Read the model definition and answer for the solid it produces. Units are mm, in the model's axes. A direction names the side the tool comes from. Coordinates: 2 decimals unless noted, no trailing zeros. Write each loop counter-clockwise with the first axis right and the second up, starting at its lowest first coordinate (ties: lowest second). Pieces come first, ordered by that corner, then holes. Notation, with made-up numbers: M 82.5,66.5 L 121.5,66.5 A18 ccw 121.5,78.5 Z; hole C 72.25,-20.5 d4. An arc over 180 degrees is marked long. Write item = value, one per line.
from build123d import *

# Parameters (mm, degrees)
BOSS_EXTRUDE1_DEPTH                           = 10
CBORE_FOR_M3_HEX_HEAD_MACHINE_SCREW3_AT_COUNT = 2
CBORE_FOR_M3_HEX_HEAD_MACHINE_SCREW3_AT_PITCH = 31.112698372
CBORE_FOR_M3_HEX_HEAD_MACHINE_SCREW3_2_COUNT  = 2
CBORE_FOR_M3_HEX_HEAD_MACHINE_SCREW3_2_PITCH  = 44


with BuildPart() as part:
    # Sketch1 → Boss-Extrude1 (new body)
    with BuildSketch(Plane.XY):
        with BuildLine():
            Line((-16.007810594, -4), (-21, -4))
            Line((-21, -4), (-21, 4))
            Line((-21, 4), (-16.007810594, 4))
            ThreePointArc((-16.007810594, 4), (0, 16.5), (16.007810594, 4))
            Line((16.007810594, 4), (24.677925359, 4))
            ThreePointArc((24.677925359, 4), (-25, 0), (24.677925359, -4))
            Line((24.677925359, -4), (16.007810594, -4))
            ThreePointArc((16.007810594, -4), (0, -16.5), (-16.007810594, -4))
        make_face()
    extrude(amount=BOSS_EXTRUDE1_DEPTH)

    # Sketch6 → CBORE for M3 Hex Head Machine Screw2 (revolve, cut)
    with BuildSketch(Plane(origin=(20.342867976, 24, 5), x_dir=(0, 0, 1), z_dir=(1, 0, 0))):
        Polygon((0, 0), (0, 49), (1.7, 49), (1.7, 17.3), (4.2, 17.3), (4.2, 0.025), (4.225, 0), align=None)
    revolve(axis=Axis((20.342867976, 30.35, 5), (0, -1, 0)), mode=Mode.SUBTRACT)

    # Sketch8 → CBORE for M3 Hex Head Machine Screw3 (revolve, cut)
    with BuildSketch(Plane(origin=(-15.556349186, 15.556349186, 10), x_dir=(0, -1, 0), z_dir=(1, 0, 0))):
        Polygon((0, 0), (0, 10), (1.7, 10), (1.7, 2.3), (4.2, 2.3), (4.2, 0.025), (4.225, 0), align=None)
    cbore_for_m3_hex_head_machine_screw3 = revolve(axis=Axis((-15.556349186, 15.556349186, 16.35), (0, 0, -1)), mode=Mode.SUBTRACT)

    # CBORE for M3 Hex Head Machine Screw3 at: CBORE for M3 Hex Head Machine Screw3 ×2
    with Locations(*[(0, -i * CBORE_FOR_M3_HEX_HEAD_MACHINE_SCREW3_AT_PITCH, 0) for i in range(1, CBORE_FOR_M3_HEX_HEAD_MACHINE_SCREW3_AT_COUNT)]):
        add(cbore_for_m3_hex_head_machine_screw3, mode=Mode.SUBTRACT)

    # CBORE for M3 Hex Head Machine Screw3 2: CBORE for M3 Hex Head Machine Screw3 ×2
    with Locations(*[Vector(0.707106781, -0.707106781, 0) * (i * CBORE_FOR_M3_HEX_HEAD_MACHINE_SCREW3_2_PITCH) for i in range(1, CBORE_FOR_M3_HEX_HEAD_MACHINE_SCREW3_2_COUNT)]):
        add(cbore_for_m3_hex_head_machine_screw3, mode=Mode.SUBTRACT)


solid = part.part
Item 1: Find section B-B (z = 5). Determine the outline of the cut face in (x, y).
Worked answers:
outline = M -21,-4 L -21,4 L -16.01,4 A16.5 cw 16.01,4 L 18.64,4 L 18.64,6.7 L 16.14,6.7 L 16.14,19.09 A25 ccw long 18.64,-16.66 L 18.64,-4 L 16.01,-4 A16.5 cw -16.01,-4 Z; M 22.04,-11.79 A25 ccw 24.68,-4 L 22.04,-4 Z; M 22.04,4 L 24.68,4 A25 ccw 24.09,6.7 L 22.04,6.7 Z; hole C -15.56,-15.56 d3.4; hole C -15.56,15.56 d3.4; hole C 15.56,-15.56 d3.4
Item 2: Flat-ended cylindrical pins translate along their axes: pin 1 (4 mm diameter, centred on x = -19, z = 4.5, fed in from -Y); pin 2 (2 mm diameter, centred on y = -11, z = 7.5, fed in from +X); pin 3 (3 mm diameter, centred on x = -5, z = 2.5, fed in from +Y). Find the tip coordinate at first contact, or state that the pin passes through.
Worked answers:
pin_1 = -18.33
pin_2 = 22.91
pin_3 = 24.75
Item 3: Which of the six approach directions +Z, -Z, +X, -X, +Y, -Y give full straight-line access (tool end or side, diameter ignored) to faces 1 (the face through (16.146, 11.605, 5.157)), 2 (the face through (-19, 4, 5)), 3 (the face through (0.306, -16.497, 4.93)), 4 (the face through (-1, 17, 0)), 5 (the face through (15.5, -13.7, 7.7))?
Worked answers:
face_1 = +Y
face_2 = +Z, -Z, +X
face_3 = +Z, -Z
face_4 = -Z, +X, -X, +Y, -Y
face_5 = +Z
Item 4: For a pull along Y with two mould halves and no side action, classify faces 6 (the face through (18.657, 5.369, 4.779)), 7 (the face through (-0.306, 16.497, 4.93)), 8 (the face through (22, 6.7, 6)) as released by +Y, released by -Y, zero draft, split by the parting line, or undercut.
Worked answers:
face_6 = zero draft
face_7 = undercut
face_8 = released by +Y
Item 5: Find section C-C (z = 2). Determine the outline of the cut face in (x, y).
Worked answers:
outline = M -21,-4 L -21,4 L -16.01,4 A16.5 cw 16.01,4 L 24.68,4 A25 ccw 23.28,9.11 L 23.28,6.7 L 17.4,6.7 L 17.4,17.95 A25 ccw long 24.68,-4 L 16.01,-4 A16.5 cw -16.01,-4 Z; hole C -15.56,-15.56 d3.4; hole C -15.56,15.56 d3.4; hole C 15.56,-15.56 d3.4
Item 6: Find section A-A (x = 0). Determine the outline of the cut face in (y, z).
Worked answers:
outline = M -25,0 L -16.5,0 L -16.5,10 L -25,10 Z; M 16.5,0 L 25,0 L 25,10 L 16.5,10 Z
Item 7: Find section D-D (x = -7.5). Determine the outline of the cut face in (y, z).
Worked answers:
outline = M -23.85,0 L -14.7,0 L -14.7,10 L -23.85,10 Z; M 14.7,0 L 23.85,0 L 23.85,10 L 14.7,10 Z
Item 8: Consider line 1 along X through (y, z) = (5.05, 5); line 2 along Z through (x, y) = (20.5, -8); line 3 along Y through (x, z) = (17, 5.5). Determine where each line is inside the solid, lowest interval first. Write a range as from..to.
Worked answers:
line_1 = -24.48..-15.71, 15.71..18.64, 22.04..24.48
line_2 = 0..3.31, 6.69..10
line_3 = -18.33..-16.45, -14.66..-4, 4..6.7
